Answer from the drawing. Dimensions are ordinates in mm from the lowest x, y and z of the part. Coordinates: 2 decimals unless noted, no trailing zeros. Write each loop counter-clockwise with the first axis right and the second up, starting at its lowest first coordinate (ties: lowest second). Pieces come first, ordered by that corner, then holes. Notation, with made-up numbers: (63.5, -27.75) -> (120.5, -27.75) arc R20 ccw to (120.5, -23.75) -> close; hole circle Ø1 at (-5, 80.25). An arc over 180 degrees is marked (long way). Return JSON: item names as keys, results as strings.
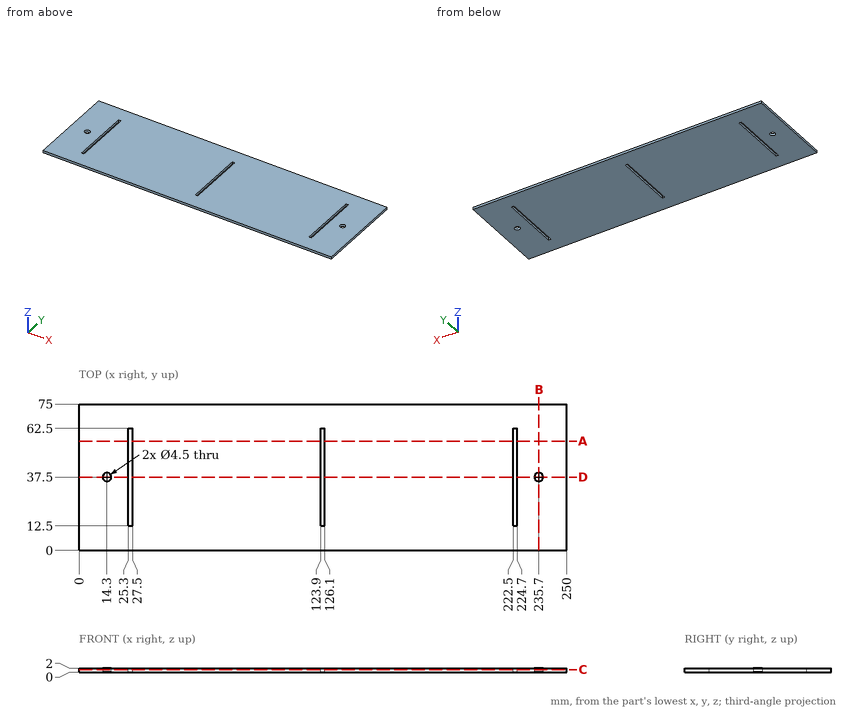
1. The part is cut by section B-B (x = 235.7). Determine the outline of the cut face in (y, z), then the cut area to 3 significant figures.
Taken from the geometry:
{"outline": "(0, 0) -> (35.25, 0) -> (35.25, 2) -> (0, 2) -> close; (39.75, 0) -> (75, 0) -> (75, 2) -> (39.75, 2) -> close", "area": "141 mm2"}
2. Consider L1, parallel to X at y = 41, z = 0.45; L2, parallel to Y at x = 235.7, z = 1.1. Determine where each line is inside the solid, lowest interval first.
Taken from the geometry:
{"L1": "x = 0 to 25.3, 27.5 to 123.9, 126.1 to 222.5, 224.7 to 250", "L2": "y = 0 to 35.25, 39.75 to 75"}
3. The part is cut by section C-C (z = 1.35). Determine the outline of the cut face in (x, y), then the cut area to 3 significant figures.
Taken from the geometry:
{"outline": "(0, 0) -> (250, 0) -> (250, 75) -> (0, 75) -> close; hole circle Ø4.5 at (14.3, 37.5); hole (25.3, 12.5) -> (27.5, 12.5) -> (27.5, 62.5) -> (25.3, 62.5) -> close; hole (123.9, 12.5) -> (126.1, 12.5) -> (126.1, 62.5) -> (123.9, 62.5) -> close; hole (222.5, 12.5) -> (224.7, 12.5) -> (224.7, 62.5) -> (222.5, 62.5) -> close; hole circle Ø4.5 at (235.7, 37.5)", "area": "18,400 mm2"}
4. The part is cut by section A-A (y = 56). Determine the outline of the cut face in (x, z), then the cut area to 3 significant figures.
Taken from the geometry:
{"outline": "(0, 0) -> (25.3, 0) -> (25.3, 2) -> (0, 2) -> close; (27.5, 0) -> (123.9, 0) -> (123.9, 2) -> (27.5, 2) -> close; (126.1, 0) -> (222.5, 0) -> (222.5, 2) -> (126.1, 2) -> close; (224.7, 0) -> (250, 0) -> (250, 2) -> (224.7, 2) -> close", "area": "487 mm2"}
5. The part is cut by section D-D (y = 37.5). Determine the outline of the cut face in (x, z).
Taken from the geometry:
{"outline": "(0, 0) -> (12.05, 0) -> (12.05, 2) -> (0, 2) -> close; (16.55, 0) -> (25.3, 0) -> (25.3, 2) -> (16.55, 2) -> close; (27.5, 0) -> (123.9, 0) -> (123.9, 2) -> (27.5, 2) -> close; (126.1, 0) -> (222.5, 0) -> (222.5, 2) -> (126.1, 2) -> close; (224.7, 0) -> (233.45, 0) -> (233.45, 2) -> (224.7, 2) -> close; (237.95, 0) -> (250, 0) -> (250, 2) -> (237.95, 2) -> close"}
